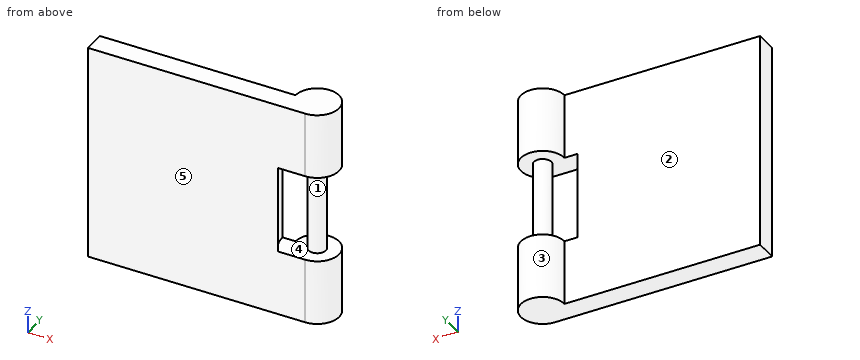
from build123d import *

# Parameters (mm, degrees)
SKETCH2_W           = 50
SKETCH2_H           = 5
BOSS_EXTRUDE1_DEPTH = 50
SKETCH3_R           = 8
CUT_EXTRUDE1_DEPTH  = 50
SKETCH4_R           = 5
BOSS_EXTRUDE2_DEPTH = 50
SKETCH6_R           = 5
CUT_EXTRUDE2_DEPTH  = 20
SKETCH7_W           = 10
SKETCH7_H           = 5
BOSS_EXTRUDE3_DEPTH = 15
LPATTERN1_COUNT     = 2
LPATTERN1_PITCH     = 35
SKETCH8_R           = 2
BOSS_EXTRUDE4_DEPTH = 50


with BuildPart() as part:
    # Sketch2 → Boss-Extrude1 (new body)
    with BuildSketch(Plane.XY):
        with Locations((-25, -2.5)):
            Rectangle(SKETCH2_W, SKETCH2_H)
    extrude(amount=-BOSS_EXTRUDE1_DEPTH)

    # Sketch3 → Cut-Extrude1 (cut)
    with BuildSketch(Plane.XY):
        Circle(SKETCH3_R)
    extrude(amount=-CUT_EXTRUDE1_DEPTH, mode=Mode.SUBTRACT)



with BuildPart() as body_2:
    # Sketch4 → Boss-Extrude2 (new body)
    with BuildSketch(Plane.XY):
        Circle(SKETCH4_R)
    extrude(amount=-BOSS_EXTRUDE2_DEPTH)

    # Sketch6 → Cut-Extrude2 (cut)
    with BuildSketch(Plane.XY.offset(-15)):
        Circle(SKETCH6_R)
    extrude(amount=-CUT_EXTRUDE2_DEPTH, mode=Mode.SUBTRACT)


with BuildPart() as cut_extrude2_piece_1:
    # of the separate pieces the step leaves, piece 1, a body of its own (cut_extrude2_pieces)
    add(body_2.part.solids().sort_by_distance((5, 0, 0))[0])


with BuildPart() as cut_extrude2_piece_2:
    # of the separate pieces the step leaves, piece 2, a body of its own (cut_extrude2_pieces)
    add(body_2.part.solids().sort_by_distance((5, 0, -35))[0])


with BuildPart() as part_1:
    add(part.part)

    add(cut_extrude2_piece_1.part)  # Boss-Extrude3 merges Cut-Extrude2 piece 1
    # Sketch7 → Boss-Extrude3 (add)
    with BuildSketch(Plane.XY):
        with Locations((-5, -2.5)):
            Rectangle(SKETCH7_W, SKETCH7_H)
    boss_extrude3 = extrude(amount=-BOSS_EXTRUDE3_DEPTH)


    add(cut_extrude2_piece_2.part)  # LPattern1 merges Cut-Extrude2 piece 2
    # LPattern1: Boss-Extrude3 ×2
    with Locations(*[(0, 0, -i * LPATTERN1_PITCH) for i in range(1, LPATTERN1_COUNT)]):
        add(boss_extrude3)

    # Sketch8 → Boss-Extrude4 (add)
    with BuildSketch(Plane.XY):
        Circle(SKETCH8_R)
    extrude(amount=-BOSS_EXTRUDE4_DEPTH)


solid = part_1.part
Geometry: final body of the model. Coordinates: model frame, mm. Face numbers are marked on the shaded views. A direction names the side the tool comes from. Round coordinates to 2 decimals unless told otherwise and drop trailing zeros. Order: outer loops, then holes, each group sorted by start corner. A loop starts at its lowest first (then second) coordinate and runs counter-clockwise, first axis right, second up. Notation, with made-up numbers: (88.5, 30) -> (145.5, 30) arc R30 ccw to (145.5, 69) -> close; hole circle Ø3 at (-9, 28.5). An arc over 180 degrees is marked (long way). Put each result on its own line as item: value. Start each with the question number.
Q1. Section D-D on x = -21.5. Return the cut outline in (y, z).
Q2. First-contact query: pin 1 (5 mm diameter, centred on x = -7.5, y = 3, fed in from +Z); pin 2 (2 mm diameter, centred on y = 2, z = -44, fed in from -X); pin 3 (10 mm diameter, centred on x = -13, z = -13.5, fed in from +Y); pin 4 (1.5 mm diameter, centred on y = 2.5, z = -27.5, fed in from +X). Flat tips, straight axial feed; report the tip coordinate or a pass-through.
Q3. Reachability of the marked faces 4 and 5 from +Z, -Z, +X, -X, +Y, -Y: full face, straight path, thin tool, end or side. Return the list, or none.
Q4. Line query: probe 1 along Z at (x, y) = (-3, 3.75); probe 2 along X at (y, z) = (-0.25, -20); probe 3 along Y at (x, z) = (-6, -41). Output: solid intervals per line, ascending.
Q5. Section B-B on y = 3.5. Return the cut outline in (x, z).
Q6. Section A-A on z = -31.5. Return the cut outline in (x, y) (3 decimals).
Q7. Pull-direction query (X, two-part tool) for the marked faces 1, 2 and 3; classes: +X half, -X half, draft (parallel to the pull), parting line (faces both ways), or undercut.
Q8. Section C-C on y = -2.75. Return the cut outline in (x, z), and give its area (3 significant figures).
Ans:
1. outline: (-5, -50) -> (0, -50) -> (0, 0) -> (-5, 0) -> close
2. pin 1: passes through
2. pin 2: stops at x = -4.9
2. pin 3: stops at y = 0
2. pin 4: stops at x = 0.97
3. face 4: none
3. face 5: +Z, -Z, +X, -X, -Y
4. probe 1: z = -50 to -35, -15 to 0
4. probe 2: x = -50 to -8, -1.98 to 1.98
4. probe 3: y = -5 to 0
5. outline: (-3.57, -50) -> (3.57, -50) -> (3.57, -35) -> (-3.57, -35) -> close; (-3.57, -15) -> (3.57, -15) -> (3.57, 0) -> (-3.57, 0) -> close
6. outline: (-50, -5) -> (-6.245, -5) arc R8 cw to (-8, 0) -> (-50, 0) -> close; circle Ø4 at (0, 0)
7. face 1: undercut
7. face 2: draft
7. face 3: parting line
8. outline: (-50, -50) -> (4.18, -50) -> (4.18, -35) -> (-7.51, -35) -> (-7.51, -15) -> (4.18, -15) -> (4.18, 0) -> (-50, 0) -> close
8. area: 2,480 mm2
